Read the model definition and answer for the solid it produces. Units are mm, in the model's axes. Coordinates: 2 decimals unless noted, no trailing zeros. Order: outer loops, then holes, each group sorted by start corner. A loop starts at its lowest first (then second) coordinate and runs counter-clockwise, first axis right, second up. Notation, with made-up numbers: (23.25, 3.25) -> (77.25, 3.25) arc R20 cw to (77.25, 42.25) -> close; hole circle Ø6 at (34, 46.5). An arc over 180 degrees is marked (long way). Use CSV: the item, a comma, the result in double quotes.
```python
from build123d import *

# Parameters (mm, degrees)
SKETCH1_R           = 10
BOSS_EXTRUDE1_DEPTH = 110
SKETCH2_R           = 6
BOSS_EXTRUDE2_DEPTH = 24
CHAMFER1_SIZE       = 2
CHAMFER2_SIZE       = 1


with BuildPart() as part:
    # Sketch1 → Boss-Extrude1 (new body)
    with BuildSketch(Plane(origin=(0, 0, 0), x_dir=(1, 0, 0), z_dir=(0, 1, 0))):
        with Locations(Location((0, 0, 0), (0, 0, 270))):
            Circle(SKETCH1_R)
    extrude(amount=BOSS_EXTRUDE1_DEPTH)

    # Sketch2 → Boss-Extrude2 (add)
    with BuildSketch(Plane(origin=(0, 110, 0), x_dir=(1, 0, 0), z_dir=(0, 1, 0))):
        with Locations(Location((0, 0, 0), (0, 0, 270))):
            Circle(SKETCH2_R)
    extrude(amount=BOSS_EXTRUDE2_DEPTH)

    # Sketch3 → Revolve1 (revolve)
    with BuildSketch(Plane(origin=(0, 0, 0), x_dir=(0, 0, -1), z_dir=(1, 0, 0))):
        with BuildLine():
            Line((0, 134), (0, 148.5))
            add(Edge.make_bspline(
                [(0, 148.5), (-3.667360113, 141.867546182), (-4, 134)],
                knots=[0, 0, 0, 1, 1, 1], degree=2))
            Line((-4, 134), (0, 134))
        make_face()
    revolve(axis=Axis((0, 134, 0), (0, -1, 0)))

    # Chamfer1
    chamfer1_edges = [part.edges().sort_by_distance(p)[0] for p in [
        (0, 134, -6),
    ]]
    chamfer(chamfer1_edges, length=CHAMFER1_SIZE - 0.0001)  # a hair under: the kernel refuses the full size

    # Chamfer2
    chamfer2_edges = [part.edges().sort_by_distance(p)[0] for p in [
        (0, 110, -10),
    ]]
    chamfer(chamfer2_edges, length=CHAMFER2_SIZE)


solid = part.part
```
Item 1: Straight lines are drawn through the part: line 1 along Y through (x, z) = (5, 3.5); line 2 along Z through (x, y) = (-0.25, 41.5); line 3 along X through (y, z) = (131.5, 0). For each, find the intervals that lie inside material, in ascending order.
Return value:
line 1,"y = 0 to 110"
line 2,"z = -10 to 10"
line 3,"x = -6 to 6"
Item 2: Find section A-A, the plane y = 67. Give the vertices of the cut face in (x, z), then the cut area to 3 significant figures.
Return value:
outline,"circle Ø20 at (0, 0)"
area,"314 mm^2"
Item 3: Each of these flat-tipped pins is pushed along its axis until it touches: P1, Ø5, axis at y = 19.5, z = 7.5, coming from the -X side; P2, Ø1.5, axis at x = 6.5, y = 133, coming from the +Z side; P3, Ø5.5, axis at x = 1, z = 4, coming from the +Y side; P4, Ø3, axis at y = 91.5, z = -6, coming from the -X side. Where does it stop, or does it pass through?
Return value:
P1,"stops at x = -8.66"
P2,"passes through"
P3,"stops at y = 145.71"
P4,"stops at x = -8.93"
Item 4: The mould has two halves that part along Y. Classify faces 1 (the flat face through (-6, 110, 2)), 2 (the cylindrical face through (1.802, 120.846, 5.723)), 3 (the flat face through (0, 0, 0)): +Y half, -Y half, draft (parallel to the pull), parting line (faces both ways), or undercut.
Return value:
face 1,"+Y half"
face 2,"draft"
face 3,"-Y half"
